CAD build for the part. Positions are in the model's coordinates, mm. Face numbers are marked on the shaded views. A direction names the side the tool comes from. Give positions to 0.01 mm unless a question says otherwise; leave off trailing zeros. Loops run counter-clockwise (first coordinate to the right, second up) from the corner with the lowest first, then second, coordinate; pieces in that order, holes last. Notation, with made-up numbers: M 35,24 L 91,24 A18 ccw 91,40 Z; hole C 63.25,-11 d8. An arc over 180 degrees is marked long. One line per question, with ' | ' between items.
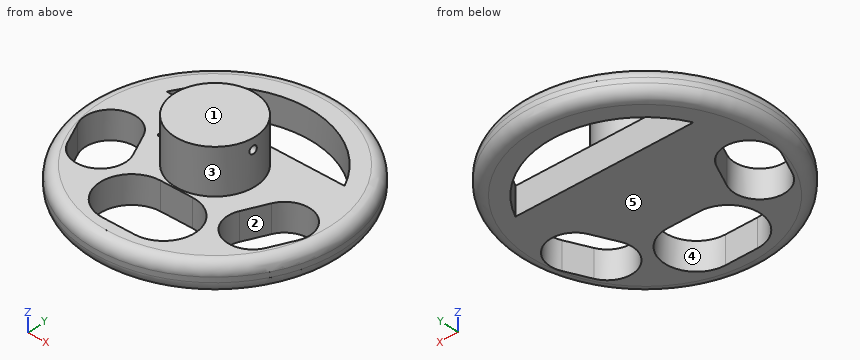
```python
from build123d import *

# Parameters (mm, degrees)
SKETCH_R     = 100
PAD_DEPTH    = 22
SKETCH001_R  = 32
PAD001_DEPTH = 35.5
SKETCH002_W  = 1
SKETCH002_H  = 1
PAD002_DEPTH = 1
SKETCH003_R  = 3
POCKET_DEPTH = 143.942083
FILLET_R     = 9


with BuildPart() as part:
    # Sketch → Pad (new body)
    with BuildSketch(Plane.XY):
        Circle(SKETCH_R)
        with BuildLine():
            Line((-70, 35), (70, 35))
            ThreePointArc((70, 35), (0, 78.262379), (-70, 35))
        make_face(mode=Mode.SUBTRACT)
        with BuildLine():
            ThreePointArc((-78.126156, -41.578521), (-51.547635, -51.252311), (-41.873844, -24.673791))
            Line((-41.873844, -24.673791), (-50.326209, -6.547635))
            ThreePointArc((-50.326209, -6.547635), (-76.90473, 3.126156), (-86.578521, -23.452365))
            Line((-78.126156, -41.578521), (-86.578521, -23.452365))
        make_face(mode=Mode.SUBTRACT)
        with BuildLine():
            ThreePointArc((41.873844, -24.673791), (51.547635, -51.252311), (78.126156, -41.578521))
            Line((78.126156, -41.578521), (86.578521, -23.452365))
            ThreePointArc((86.578521, -23.452365), (76.90473, 3.126156), (50.326209, -6.547635))
            Line((41.873844, -24.673791), (50.326209, -6.547635))
        make_face(mode=Mode.SUBTRACT)
        with BuildLine():
            Line((12.5, -33.126156), (-12.5, -33.126156))
            ThreePointArc((-12.5, -33.126156), (-37.5, -58.126156), (-12.5, -83.126156))
            Line((12.5, -83.126156), (-12.5, -83.126156))
            ThreePointArc((12.5, -83.126156), (37.5, -58.126156), (12.5, -33.126156))
        make_face(mode=Mode.SUBTRACT)
    extrude(amount=PAD_DEPTH)

    # Sketch001 → Pad001 (new body)
    with BuildSketch(Plane.XY.offset(22)):
        Circle(SKETCH001_R)
    extrude(amount=PAD001_DEPTH)

    # Sketch002 → Pad002 (new body)
    with BuildSketch(Plane.XY.offset(22)):
        with Locations((-43.441083, -0.5)):
            Rectangle(SKETCH002_W, SKETCH002_H)
    extrude(amount=PAD002_DEPTH)

    # Sketch003 → Pocket (cut, through all)
    with BuildSketch(Plane(origin=(-43.941083, 0, 0), x_dir=(0, -1, 0), z_dir=(-1, 0, 0))):
        with Locations((2, 49)):
            Circle(SKETCH003_R)
    extrude(amount=-POCKET_DEPTH, mode=Mode.SUBTRACT)

    # Fillet
    fillet_edges = [part.edges().sort_by_distance(p)[0] for p in [
        (-100, 0, 22),
        (-100, 0, 0),
    ]]
    fillet(fillet_edges, radius=FILLET_R)


solid = part.part
```
Item 1: Mould opens along X. For the marked faces 3, 4 and 5 say: pulls with the +X half, pulls with the -X half, needs draft (parallel to the pull), parting line crosses it, or undercut.
Conclusion:
face 3: parting line crosses it | face 4: undercut | face 5: needs draft
Item 2: 3-axis set-ups, long thin cutter, end or side, ignore diameter. For the marked faces 1 and 2: which of +Z, -Z, +X, -X, +Y, -Y reach the whole face in a straight line?
Conclusion:
face 1: +Z, +X, -X, +Y, -Y | face 2: +Z, -Z
Item 3: Saw through at B-B on x = -8. State how many separate pieces and enclosed holes the cut face has, and give its area (3 significant figures).
Conclusion:
separate pieces: 3 | enclosed holes: 1 | area: 4,440 mm²
Item 4: Drill centre lines: line 1 along Z through (x, y) = (11.5, -2); line 2 along Y through (x, z) = (67.5, 7); line 3 along X through (y, z) = (70, 16). Where is each one in solid material? Low to high. Write a range as [from, to].
Conclusion:
line 1: [0, 46], [52, 57.5] | line 2: [-73.48, -51.67], [4.98, 35], [39.61, 73.48] | line 3: [-70.69, -35], [35, 70.69]
Item 5: Saw through at A-A on z = 37.5. Give the cut face in (x, y).
Conclusion:
outline: C 0,0 d64
Item 6: Drop flat-ended pins along their axis: P1, Ø1.1, axis at x = -43.5, y = -0.5, coming from the +Z side; P2, Ø0.5, axis at y = -0.5, z = 22.5, coming from the -X side; P3, Ø9.5, axis at y = -2, z = 49, coming from the -X side. Give the stop position or say it passes through.
Conclusion:
P1: z = 23 | P2: x = -43.94 | P3: x = -32
